Input: part model. Units: mm. Frame: model coordinates. Coordinates: 2 decimals unless noted, no trailing zeros. Loops run counter-clockwise (first coordinate to the right, second up) from the corner with the lowest first, then second, coordinate; pieces in that order, holes last. Notation, with made-up numbers: (37.25, 46) - (77.25, 46) arc R33 cw to (77.25, 74) - close; hole circle Ø9 at (79, 22.5). An arc over 180 degrees is marked (long way). Use a Markdown table: item, result. Add a question column.
1. Contact query for flat-ended pins moving along their axis: P1, Ø1.5, axis at x = 62.5, z = 1, coming from the -Y side; P2, Ø1, axis at y = -28.5, z = 2.5, coming from the -X side. Output: stop coordinate, or through.
2. Section query B-B on y = -16.5. Return the cut outline in (x, z).
3. Section query A-A on z = 2.1. Return the cut outline in (x, y), then the cut area to 3 significant figures.
4. Ray query, L1, parallel to Y at x = 28.5, z = 2.2; L2, parallel to X at y = -10, z = 1.3; L3, parallel to Y at x = 26.5, z = 1.5. Return the intervals inside material, ascending. Write a range as [from, to].
5. Section query C-C on x = 50.5. Return the cut outline in (y, z).
```python
from build123d import *

# Parameters (mm, degrees)
BOSS_EXTRUDE1_START     = -3
BOSS_EXTRUDE1_OUTLINE_R = 2.5
BOSS_EXTRUDE1_DEPTH     = 3
FILLET1_R               = 10
BOSS_EXTRUDE2_START     = -3
BOSS_EXTRUDE2_DEPTH     = 3
CUT_EXTRUDE1_START      = -3
CUT_EXTRUDE1_DEPTH      = 3
FILLET2_R               = 10
CUT_EXTRUDE2_DEPTH      = 103.947966144
CUT_EXTRUDE2_DEPTH_BACK = 103.947966144


with BuildPart() as part:
    # Boss-Extrude1: read off the stored shape, not the designer's step
    # Boss-Extrude1 outline → Boss-Extrude1 (new body)
    with BuildSketch(Plane.XY.offset(3).offset(BOSS_EXTRUDE1_START)):
        with BuildLine():
            ThreePointArc((-24.364065342, 16.876742294), (-25.101814907, 17.696096192), (-26.161653435, 18))
            Line((-26.161653435, 18), (-27.830556346, 18))
            ThreePointArc((-27.830556346, 18), (-29.526652538, 17.059838528), (-29.628144438, 15.123257706))
            Line((-29.628144438, 15.123257706), (-16.550964109, -11.68893536))
            ThreePointArc((-16.550964109, -11.68893536), (-15.603505287, -14.937815984), (-15.793938159, -18.316667689))
            Line((-15.793938159, -18.316667689), (-24.617449619, -56.633968709))
            ThreePointArc((-24.617449619, -56.633968709), (-12.550978841, -74.781492041), (4.900124379, -61.728089553))
            Line((4.900124379, -61.728089553), (7.520756747, -39.132184047))
            Line((7.520756747, -39.132184047), (57.484416951, -6.361887987))
            ThreePointArc((57.484416951, -6.361887987), (61.581724267, 4.861915454), (52, 12))
            Line((52, 12), (41.720733512, 12))
            ThreePointArc((41.720733512, 12), (27.868275115, 8.610324995), (17.146172183, -0.792706909))
            Line((17.146172183, -0.792706909), (11.877704642, -8.316858327))
            ThreePointArc((11.877704642, -8.316858327), (-1.137656888, -14.455301339), (-13.032513671, -6.356381628))
            Line((-13.032513671, -6.356381628), (-24.364065342, 16.876742294))
        make_face()
        with Locations((-10, -60)):
            Circle(BOSS_EXTRUDE1_OUTLINE_R, mode=Mode.SUBTRACT)
    extrude(amount=BOSS_EXTRUDE1_DEPTH)

    # Fillet1
    fillet1_edges = [part.edges().sort_by_distance(p)[0] for p in [
        (7.520756747, -39.132184047, 1.5),
    ]]
    fillet(fillet1_edges, radius=FILLET1_R)

    # Sketch2 → Boss-Extrude2 (add)
    with BuildSketch(Plane.XY.offset(3).offset(BOSS_EXTRUDE2_START)):
        with BuildLine():
            Line((11.431019345, -36.567510792), (71.720733512, -18))
            ThreePointArc((71.720733512, -18), (69.105682696, -5.749915992), (61.716429632, 4.364528537))
            ThreePointArc((61.716429632, 4.364528537), (61.302173782, -1.670090316), (57.484416951, -6.361887987))
            Line((57.484416951, -6.361887987), (11.431019345, -36.567510792))
        make_face()
    extrude(amount=BOSS_EXTRUDE2_DEPTH)

    # Sketch2<4> → Cut-Extrude1 (cut)
    with BuildSketch(Plane.XY.offset(3).offset(CUT_EXTRUDE1_START)):
        with BuildLine():
            ThreePointArc((41.720733512, 12), (52.42269931, 10.026200742), (61.716429632, 4.364528537))
            ThreePointArc((61.716429632, 4.364528537), (58.178782835, 9.862737607), (52, 12))
            Line((52, 12), (41.720733512, 12))
        make_face()
    extrude(amount=CUT_EXTRUDE1_DEPTH, mode=Mode.SUBTRACT)

    # Fillet2
    fillet2_edges = [part.edges().sort_by_distance(p)[0] for p in [
        (71.720733512, -18, 1.5),
    ]]
    fillet(fillet2_edges, radius=FILLET2_R)

    # Sketch3 → Cut-Extrude2 (cut, two sides: drawn at the far end of the back side and taken through both)
    with BuildSketch(Plane.XY.offset(3).offset(-CUT_EXTRUDE2_DEPTH_BACK)):
        Polygon((-108.405592733, 346.786455555), (-15.36308768, 49.146087288), (29.942477709, -95.785147736), (122.984982762, -393.425516003), (-472.295753771, -579.510526109), (-703.686329267, 160.701445449), align=None)
    extrude(amount=CUT_EXTRUDE2_DEPTH + CUT_EXTRUDE2_DEPTH_BACK, mode=Mode.SUBTRACT)


solid = part.part
```
Resolved:
| question | item | result |
|---|---|---|
| 1 | P1 | y = -21.07 |
| 1 | P2 | x = 8.75 |
| 2 | outline | (5.16, 0) - (68.81, 0) - (68.81, 3) - (5.16, 3) - close |
| 3 | outline | (4.33, -13.84) - (11.43, -36.57) - (63.4, -20.56) arc R10 ccw to (69.83, -7.51) arc R30 ccw to (17.15, -0.79) - (11.88, -8.32) arc R14.5 cw to start |
| 3 | area | 2,060 mm² |
| 4 | L1 | [-31.31, 8.93] |
| 4 | L2 | [10.5, 70.41] |
| 4 | L3 | [-31.93, 7.85] |
| 5 | outline | (-24.54, 0) - (10.69, 0) - (10.69, 3) - (-24.54, 3) - close |
